Input: part model. Units: mm. Frame: model coordinates. A direction names the side the tool comes from. Give positions to 0.01 mm unless a question says otherwise; leave off trailing zeros. Loops run counter-clockwise (first coordinate to the right, second up) from the corner with the lowest first, then second, coordinate; pieces in that order, holes last. Notation, with made-up numbers: M 13.5,22.25 L 64.5,22.25 A21 ccw 64.5,34.25 Z; hole C 32.5,-16.5 d7. An arc over 180 degrees is marked long. One line per item, written item: value. Start each with the question number.
(1) Ray query, line 1 along Y through (x, z) = (-28.5, 30); line 2 along Z through (x, y) = (-81, 76); line 3 along X through (y, z) = (710, 42). Return the intervals inside material, ascending. Write a range as from..to.
(2) Section C-C on y = -76.2. Output: boundary loops of the cut face in (x, z) (3 decimals).
(3) Access query for faces 1 (the flat face through (-101.6, 491, 25)), 2 (the flat face through (-1, -25.4, 25)), 3 (the flat face through (-1, 1041.4, 25)). Directions: +Z, -Z, +X, -X, +Y, -Y. A direction counts if a zero-diameter tool reaches every point of the face in a straight line with its end or side. Return the directions, or none.
(4) Section B-B on x = 5.5. Output: boundary loops of the cut face in (y, z).
(5) Pull-direction query (Y, two-part tool) for faces 4 (the cylindrical face through (89.08, -60.46, 27.47)), 5 (the flat face through (89, -101.6, 25)), 6 (the flat face through (-76.2, -56, 25)), 7 (the cylindrical face through (-88.72, -60.46, 27.47)); classes: released by +Y, released by -Y, zero draft, split by the parting line, or undercut.
(6) Section A-A on y = 688. Output: boundary loops of the cut face in (x, z), plus the area to 3 significant figures.
(7) Pin query (flat end, axial travel): P1, Ø1.5, axis at x = 72, z = 21, coming from the -Y side. Return the tip coordinate at first contact, or that it passes through.
```python
from build123d import *

# Parameters (mm, degrees)
SKETCH1_W           = 152.4
SKETCH1_H           = 1016
BOSS_EXTRUDE1_DEPTH = 50.8
SKETCH2_R           = 15.875
SKETCH2_R_2         = 6.35
CUT_EXTRUDE1_DEPTH  = 1088.167475599


with BuildPart() as part:
    # Sketch1 → Boss-Extrude1 (new body)
    with BuildSketch(Plane.XY):
        Polygon((-76.2, -25.4), (76.2, -25.4), (76.2, -101.6), (101.6, -101.6), (101.6, 1066.8), (-101.6, 1066.8), (-101.6, -101.6), (-76.2, -101.6), align=None)
        with Locations((0, 533.4)):
            Rectangle(SKETCH1_W, SKETCH1_H, mode=Mode.SUBTRACT)
    extrude(amount=BOSS_EXTRUDE1_DEPTH)

    # Sketch2 → Cut-Extrude1 (cut, through all)
    with BuildSketch(Plane(origin=(101.6, 0, 0), x_dir=(0, 0, -1), z_dir=(1, 0, 0))):
        with Locations((-25.4, -76.2)):
            Circle(SKETCH2_R)
        with Locations((-25.4, 76.2)):
            Circle(SKETCH2_R_2)
    extrude(amount=-CUT_EXTRUDE1_DEPTH, mode=Mode.SUBTRACT)


solid = part.part
```
Output values:
1. line 1: y = -25.4..25.4, 1041.4..1066.8
1. line 2: z = 0..19.05, 31.75..50.8
1. line 3: x = -101.6..-76.2, 76.2..101.6
2. outline: M -101.6,0 L -76.2,0 L -76.2,9.525 L -101.6,9.525 Z; M -101.6,41.275 L -76.2,41.275 L -76.2,50.8 L -101.6,50.8 Z; M 76.2,0 L 101.6,0 L 101.6,9.525 L 76.2,9.525 Z; M 76.2,41.275 L 101.6,41.275 L 101.6,50.8 L 76.2,50.8 Z
3. face 1: +Z, -Z, -X, +Y, -Y
3. face 2: +Z, -Z, -Y
3. face 3: +Z, -Z
4. outline: M -25.4,0 L 25.4,0 L 25.4,50.8 L -25.4,50.8 Z; M 1041.4,0 L 1066.8,0 L 1066.8,50.8 L 1041.4,50.8 Z
5. face 4: undercut
5. face 5: released by -Y
5. face 6: zero draft
5. face 7: undercut
6. outline: M -101.6,0 L -76.2,0 L -76.2,50.8 L -101.6,50.8 Z; M 76.2,0 L 101.6,0 L 101.6,50.8 L 76.2,50.8 Z
6. area: 2,580 mm²
7. P1: stops at y = -25.4
